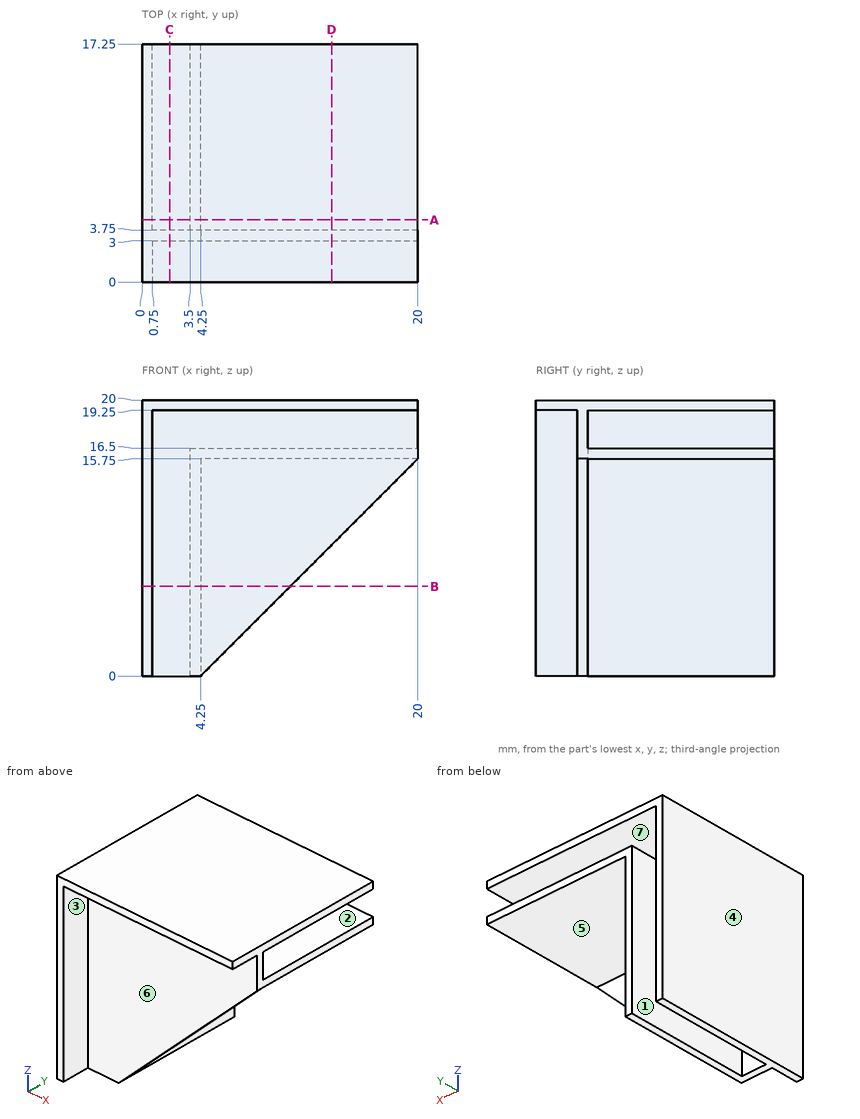
Check sheet for the drawn part. Datum: minimum x, y, z corner. Units: mm. A direction names the side the tool comes from. Coordinates: 2 decimals unless noted, no trailing zeros. Write each loop counter-clockwise with the first axis right and the second up, starting at its lowest first coordinate (ties: lowest second). Pieces come first, ordered by that corner, then holes. Notation, with made-up numbers: (26, 60) - (46, 60) arc R12 cw to (46, 78) - close; hole circle Ø10 at (-36, -13.5). An arc over 180 degrees is marked (long way). Answer as a JSON object with one key per item and string values.
(1) Gauge pin test, flat ends, axial feed: pin 1 Ø6 at (x, z) = (16, 3.5) entering from -Y; pin 2 Ø0.9 at (x, y) = (12, 1) entering from -Z; pin 3 Ø9.5 at (x, z) = (10.5, 5) entering from -Y; pin 4 Ø4 at (x, y) = (9.5, 8) entering from -Z. Record the tip position at first contact, or that the pin passes through.
Report:
{"pin 1": "through", "pin 2": "z = 19.25", "pin 3": "y = 3", "pin 4": "z = 15.75"}
(2) Tool access check on the marked faces 4, 5, 6 and 7. Record the directions out of +Z, -Z, +X, -X, +Y, -Y that give a thin tool (end or side, any length) a straight path to the whole face; none if there is none.
Report:
{"face 4": "+Z, -Z, -X, +Y, -Y", "face 5": "-Z, +X, +Y", "face 6": "-Z, +X, -Y", "face 7": "+X, +Y"}
(3) Cross-section at C-C on x = 2. Record the cut outline in (y, z), plus the area to 3 significant figures.
Report:
{"outline": "(0, 19.25) - (3, 19.25) - (3, 0) - (3.75, 0) - (3.75, 19.25) - (17.25, 19.25) - (17.25, 20) - (0, 20) - close", "area": "27.4 mm^2"}
(4) Cross-section at B-B on z = 6.5. Record the cut outline in (x, y), plus the area to 3 significant figures.
Report:
{"outline": "(0, 0) - (0.75, 0) - (0.75, 3) - (10.75, 3) - (10.75, 3.75) - (4.25, 3.75) - (4.25, 17.25) - (3.5, 17.25) - (3.5, 3.75) - (0.75, 3.75) - (0.75, 17.25) - (0, 17.25) - close", "area": "30.6 mm^2"}
(5) Cross-section at D-D on x = 13.75. Record the cut outline in (y, z).
Report:
{"outline": "(0, 19.25) - (3, 19.25) - (3, 9.5) - (3.75, 9.5) - (3.75, 15.75) - (17.25, 15.75) - (17.25, 16.5) - (3.75, 16.5) - (3.75, 19.25) - (17.25, 19.25) - (17.25, 20) - (0, 20) - close"}
(6) Cross-section at A-A on y = 4.5. Record the cut outline in (x, z).
Report:
{"outline": "(0, 0) - (0.75, 0) - (0.75, 19.25) - (20, 19.25) - (20, 20) - (0, 20) - close; (3.5, 0) - (4.25, 0) - (4.25, 15.75) - (20, 15.75) - (20, 16.5) - (3.5, 16.5) - close"}
(7) Thickness scan on line 1 along Z through (x, y) = (4, 15); line 2 along Z through (x, y) = (17.25, 6); line 3 along X through (y, z) = (7.25, 12.75). Record the ranges inside material, lowest first.
Report:
{"line 1": "0 to 16.5, 19.25 to 20", "line 2": "15.75 to 16.5, 19.25 to 20", "line 3": "0 to 0.75, 3.5 to 4.25"}
(8) Mould release check, pull along X, two halves, no side actions. Record for the marked faces 1, 2 and 3: pulls with the +X half, pulls with the -X half, needs draft (parallel to the pull), parting line crosses it, or undercut.
Report:
{"face 1": "undercut", "face 2": "needs draft", "face 3": "pulls with the +X half"}
